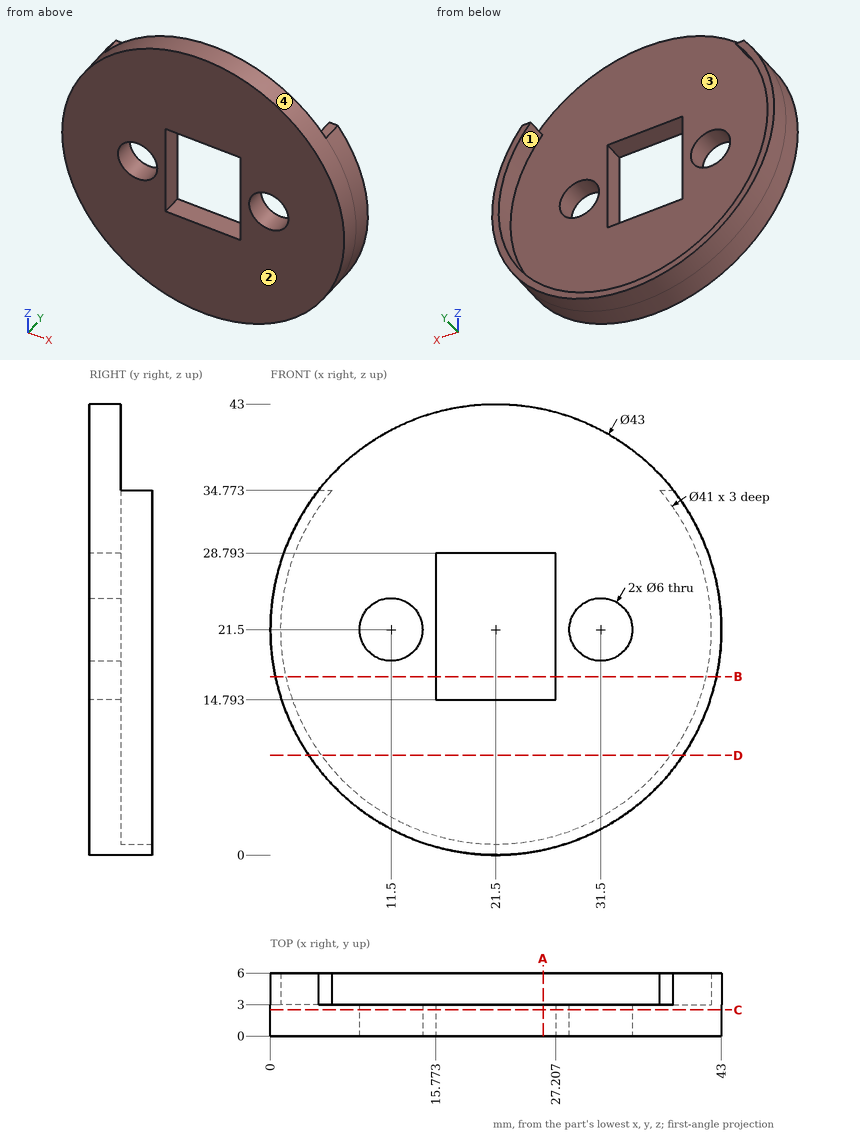
Geometry: see drawing. Coordinates: mm, zero at the bounding-box minimum. Give positions to 0.01 mm unless a question says otherwise; leave off trailing zeros. Write each loop counter-clockwise with the first axis right and the second up, starting at its lowest first coordinate (ties: lowest second). Pieces come first, ordered by that corner, then holes. Notation, with made-up numbers: M 73,56.5 L 131,56.5 A12 cw 131,67.5 Z; hole C 4.5,65.5 d10. An arc over 180 degrees is marked long. Return JSON: item names as keys, results as strings. Group by question number.
1) Ray query, L1, parallel to Y at x = 11, z = 13; L2, parallel to Z at x = 11, y = 2.5; L3, parallel to X at y = 3.5, z = 3 (1 decimal). Return the intervals inside material, ascending.
2) First-contact query: pin 1 Ø1.5 at (x, z) = (32.5, 6.5) entering from +Y; pin 2 Ø2.5 at (y, z) = (2, 23) entering from +X; pin 3 Ø0.6 at (x, y) = (37.5, 4) entering from +Z. Flat tips, straight axial feed; report the tip coordinate or a pass-through.
3) Cut plane B-B, the plane z = 17. Output: boundary loops of the cut face in (x, y).
4) Cut plane D-D, the plane z = 9.5. Output: boundary loops of the cut face in (x, y), then the cut area to 3 significant figures.
5) Draft query along Z for the marked faces 1, 2, 3 and 4. Return one class per face: released by +Z, released by -Z, zero draft, split by the parting line, or undercut.
6) Cut plane A-A, the plane x = 26. Output: boundary loops of the cut face in (y, z), then the cut area to 3 significant figures.
7) Cut plane C-C, the plane y = 2.5. Output: boundary loops of the cut face in (x, z).
Data:
{
 "1": {"L1": "y = 0 to 3", "L2": "z = 2.74 to 18.54, 24.46 to 40.26", "L3": "x = 10.5 to 12.7, 30.3 to 32.5"},
 "2": {"pin 1": "stops at y = 3", "pin 2": "stops at x = 43", "pin 3": "stops at z = 34.77"},
 "3": {"outline": "M 0.48,0 L 15.77,0 L 15.77,3 L 1.5,3 L 1.5,6 L 0.48,6 Z; M 27.21,0 L 42.52,0 L 42.52,6 L 41.5,6 L 41.5,3 L 27.21,3 Z"},
 "4": {"outline": "M 3.66,0 L 39.34,0 L 39.34,6 L 38.12,6 L 38.12,3 L 4.88,3 L 4.88,6 L 3.66,6 Z", "area": "114 mm²"},
 "5": {"face 1": "undercut", "face 2": "zero draft", "face 3": "undercut", "face 4": "split by the parting line"},
 "6": {"outline": "M 0,0.48 L 6,0.48 L 6,1.5 L 3,1.5 L 3,14.79 L 0,14.79 Z; M 0,28.79 L 3,28.79 L 3,42.52 L 0,42.52 Z", "area": "87.2 mm²"},
 "7": {"outline": "C 21.5,21.5 d43; hole C 11.5,21.5 d6; hole M 15.77,14.79 L 27.21,14.79 L 27.21,28.79 L 15.77,28.79 Z; hole C 31.5,21.5 d6"}
}
